Job drawing, mm, ordinate dimensions from the low corner. One solid piece. Round coordinates to 2 decimals unless told otherwise and drop trailing zeros. Write each loop counter-clockwise with the first axis right and the second up, starting at its lowest first coordinate (ties: lowest second). Pieces come first, ordered by that corner, then holes.
1) Saw through at B-B (y = 2.75). Write the cut outline in (x, z), plus the area to 3 significant figures.
2) Wall check: probe 1 along Z at (x, y) = (9, 0.65); probe 2 along Z at (x, y) = (14, 3). Give the ranges that are in metal, low to high.
3) Saw through at D-D (z = 6.5). Write the cut outline in (x, y).
4) Flat gauge pin, fed straight in: pin 1 (1.5 mm diameter, centred on x = 32.5, z = 6.5, fed in from +Y). Where does the tip first touch, or does it go through?
5) Saw through at C-C (x = 13). Write the cut outline in (y, z).
6) Saw through at A-A (z = 21). Write the cut outline in (x, y), plus the area to 3 significant figures.
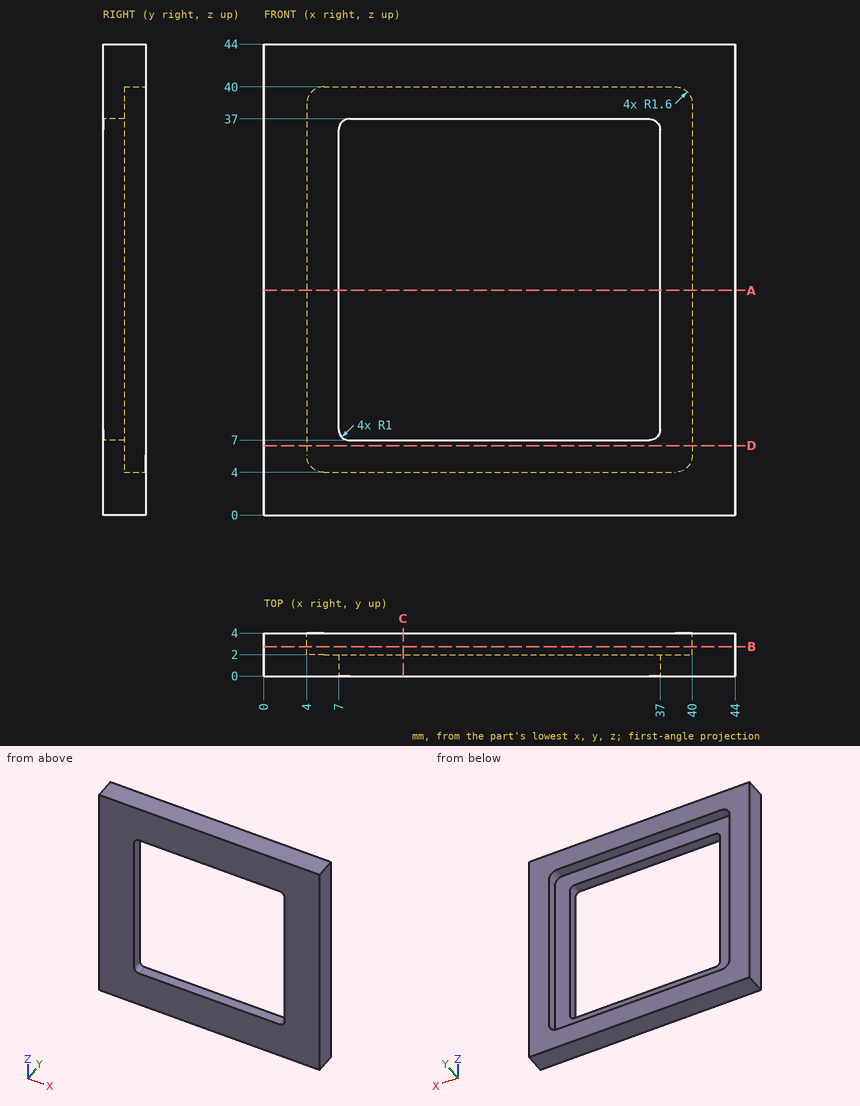
Evaluation:
1. outline: (0, 0) - (44, 0) - (44, 44) - (0, 44) - close; hole (4, 5.6) arc R1.6 ccw to (5.6, 4) - (38.4, 4) arc R1.6 ccw to (40, 5.6) - (40, 38.4) arc R1.6 ccw to (38.4, 40) - (5.6, 40) arc R1.6 ccw to (4, 38.4) - close
1. area: 642 mm2
2. probe 1: z = 0 to 7, 37 to 44
2. probe 2: z = 0 to 4, 40 to 44
3. outline: (0, 0) - (44, 0) - (44, 4) - (40, 4) - (40, 2) - (4, 2) - (4, 4) - (0, 4) - close
4. pin 1: stops at y = 2
5. outline: (0, 0) - (4, 0) - (4, 4) - (2, 4) - (2, 7) - (0, 7) - close; (0, 37) - (2, 37) - (2, 40) - (4, 40) - (4, 44) - (0, 44) - close
6. outline: (0, 0) - (7, 0) - (7, 2) - (4, 2) - (4, 4) - (0, 4) - close; (37, 0) - (44, 0) - (44, 4) - (40, 4) - (40, 2) - (37, 2) - close
6. area: 44.0 mm2
